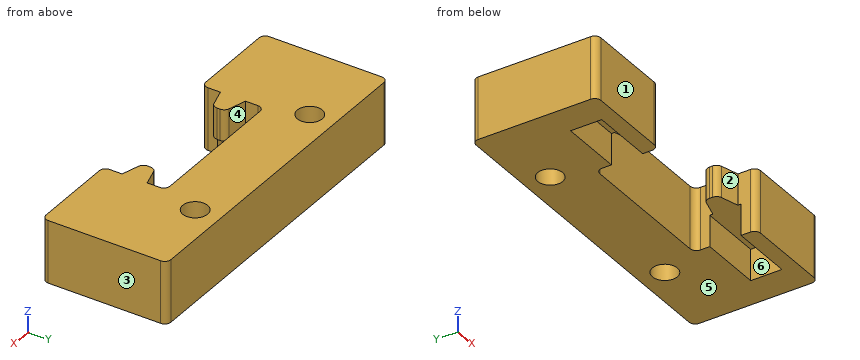
from build123d import *

# Parameters (mm, degrees)
BOSS_EXTRUDE1_DEPTH   = 5
CHAMFER1_SIZE         = 0.5
CHAMFER1_SIZE2        = 1.743707222
CHAMFER1_PART_2_SIZE  = 0.5
CHAMFER1_PART_2_SIZE2 = 1.743707222
FILLET1_R             = 0.5
SKETCH2_R             = 1
CUT_EXTRUDE1_DEPTH    = 5
FILLET2_R             = 0.5
SKETCH4_W             = 6.75
SKETCH4_H             = 2.5
CUT_EXTRUDE2_DEPTH    = 2.5


with BuildPart() as part:
    # Sketch1 → Boss-Extrude1 (new body)
    with BuildSketch(Plane.XY):
        Polygon((-6, -1.5), (-6, 0), (6, 0), (6, -1.5), (4.25, -1.5), (4.25, -3.5), (6, -3.5), (6, -5), (13.5, -5), (13.5, 5), (-13.5, 5), (-13.5, -5), (-6, -5), (-6, -3.5), (-4.25, -3.5), (-4.25, -1.5), align=None)
    extrude(amount=BOSS_EXTRUDE1_DEPTH)

    # Chamfer1
    chamfer1_edges = [part.edges().sort_by_distance(p)[0] for p in [
        (4.25, -3.5, 2.5),
        (4.25, -1.5, 2.5),
    ]]
    chamfer1_side = [part.faces().sort_by_distance(p)[0] for p in [
        (4.25, -2.5, 2.5),
    ]]
    chamfer(chamfer1_edges, length=CHAMFER1_SIZE, length2=CHAMFER1_SIZE2, reference=chamfer1_side[0])

    # Chamfer1 part 2
    chamfer1_part_2_edges = [part.edges().sort_by_distance(p)[0] for p in [
        (-4.25, -1.5, 2.5),
        (-4.25, -3.5, 2.5),
    ]]
    chamfer1_part_2_side = [part.faces().sort_by_distance(p)[0] for p in [
        (-4.25, -2.5, 2.5),
    ]]
    chamfer(chamfer1_part_2_edges, length=CHAMFER1_PART_2_SIZE, length2=CHAMFER1_PART_2_SIZE2, reference=chamfer1_part_2_side[0])

    # Fillet1
    fillet1_edges = [part.edges().sort_by_distance(p)[0] for p in [
        (4.25, -2, 2.5),
        (4.25, -3, 2.5),
        (-4.25, -2, 2.5),
        (-4.25, -3, 2.5),
    ]]
    fillet(fillet1_edges, radius=FILLET1_R)

    # Sketch2 → Cut-Extrude1 (cut)
    with BuildSketch(Plane.XY.offset(5)):
        with Locations((-7, 3)):
            Circle(SKETCH2_R)
        with Locations((7, 3)):
            Circle(SKETCH2_R)
    extrude(amount=-CUT_EXTRUDE1_DEPTH, mode=Mode.SUBTRACT)

    # Fillet2
    fillet2_edges = [part.edges().sort_by_distance(p)[0] for p in [
        (6, -5, 2.5),
        (6, 0, 2.5),
        (-6, 0, 2.5),
        (-6, -5, 2.5),
        (-13.5, -5, 2.5),
        (-13.5, 5, 2.5),
        (13.5, 5, 2.5),
        (13.5, -5, 2.5),
    ]]
    fillet(fillet2_edges, radius=FILLET2_R)

    # Sketch4 → Cut-Extrude2 (cut)
    with BuildSketch(Plane(origin=(0, 0, 0), x_dir=(-1, 0, 0), z_dir=(0, 0, -1))):
        with Locations((-7.625, -2.5)):
            Rectangle(SKETCH4_W, SKETCH4_H)
        with Locations((7.625, -2.5)):
            Rectangle(SKETCH4_W, SKETCH4_H)
    extrude(amount=-CUT_EXTRUDE2_DEPTH, mode=Mode.SUBTRACT)


solid = part.part
Input: part model. Units: mm. Frame: model coordinates. Face numbers are marked on the shaded views. A direction names the side the tool comes from. Give positions to 0.01 mm unless a question says otherwise; leave off trailing zeros. Order: outer loops, then holes, each group sorted by start corner. A loop starts at its lowest first (then second) coordinate and runs counter-clockwise, first axis right, second up. Notation, with made-up numbers: (58, 2.25) -> (114, 2.25) arc R24 cw to (114, 41.25) -> close; hole circle Ø1 at (42.5, 25.5). An arc over 180 degrees is marked (long way). Use one line per item in the form item = value.
1) Reachability of the marked faces 5 and 6 from +Z, -Z, +X, -X, +Y, -Y: full face, straight path, thin tool, end or side. Return the list, or none.
Response values:
face_5 = -Z, +X, -X, +Y, -Y
face_6 = -Z
2) First-contact query: pin 1 Ø2 at (x, y) = (-6, -2.5) entering from -Z. Flat tip, straight axial feed; report the tip coordinate or a pass-through.
Response values:
pin_1 = 2.5
3) Section B-B, the plane x = 7. Return loops of the section in (y, z).
Response values:
outline = (-5, 0) -> (-3.75, 0) -> (-3.75, 2.5) -> (-1.25, 2.5) -> (-1.25, 0) -> (2, 0) -> (2, 5) -> (-5, 5) -> close; (4, 0) -> (5, 0) -> (5, 5) -> (4, 5) -> close
4) Line query: probe 1 along Y at (x, z) = (7, 3.7); probe 2 along Y at (x, z) = (-10.25, 1.2); probe 3 along Y at (x, z) = (7.75, 1.35). Output: solid intervals per line, ascending.
Response values:
probe_1 = -5 to 2, 4 to 5
probe_2 = -5 to -3.75, -1.25 to 5
probe_3 = -5 to -3.75, -1.25 to 2.34, 3.66 to 5
5) Section A-A, the plane z = 1.75. Return loops of the section in (x, y), and give its area (3 significant figures).
Response values:
outline = (-13.5, -4.5) arc R0.5 ccw to (-13, -5) -> (-6.5, -5) arc R0.5 ccw to (-6, -4.5) -> (-6, -3.75) -> (-11, -3.75) -> (-11, -1.25) -> (-6, -1.25) -> (-6, -0.5) arc R0.5 cw to (-5.5, 0) -> (5.5, 0) arc R0.5 cw to (6, -0.5) -> (6, -1.25) -> (11, -1.25) -> (11, -3.75) -> (6, -3.75) -> (6, -4.5) arc R0.5 ccw to (6.5, -5) -> (13, -5) arc R0.5 ccw to (13.5, -4.5) -> (13.5, 4.5) arc R0.5 ccw to (13, 5) -> (-13, 5) arc R0.5 ccw to (-13.5, 4.5) -> close; hole circle Ø2 at (-7, 3); hole circle Ø2 at (7, 3)
area = 179 mm^2
6) Section C-C, the plane y = 2.75. Return loops of the section in (x, z), and give its area (3 significant figures).
Response values:
outline = (-13.5, 0) -> (-7.97, 0) -> (-7.97, 5) -> (-13.5, 5) -> close; (-6.03, 0) -> (6.03, 0) -> (6.03, 5) -> (-6.03, 5) -> close; (7.97, 0) -> (13.5, 0) -> (13.5, 5) -> (7.97, 5) -> close
area = 116 mm^2
7) Mould query, pull axis X, two halves, no side actions, for the marked faces 1, 2, 3 and 4. Classes: pulls with the +X half, pulls with the -X half, needs draft (parallel to the pull), parting line crosses it, or undercut.
Response values:
face_1 = needs draft
face_2 = undercut
face_3 = pulls with the +X half
face_4 = undercut
8) Section D-D, the plane z = 4.15. Count the separate pieces of the cut face and the enclosed holes in it, and give its area (3 significant figures).
Response values:
separate_pieces = 1
enclosed_holes = 2
area = 209 mm^2
